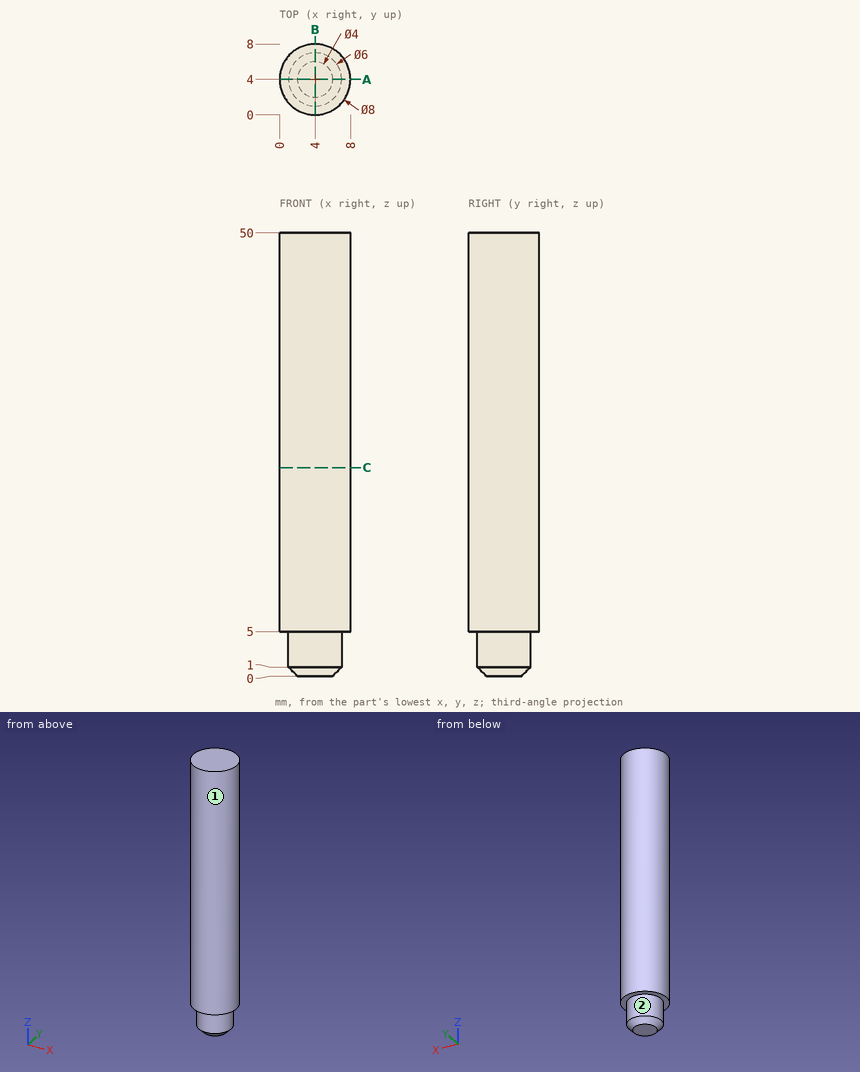
Geometry: see drawing. Coordinates: mm, zero at the bounding-box minimum. A direction names the side the tool comes from. Coordinates: 2 decimals unless noted, no trailing zeros. Loops run counter-clockwise (first coordinate to the right, second up) from the corner with the lowest first, then second, coordinate; pieces in that order, holes last. Notation, with made-up numbers: (-6.5, 33) - (32.5, 33) arc R24 ccw to (32.5, 48) - close; hole circle Ø9 at (-32, -3). An arc over 180 degrees is marked (long way). Put each result on its own line as item: value. Start each with the question number.
Q1. Set-up query: the marked faces 1 and 2. Return all of +Z, -Z, +X, -X, +Y, -Y with unobstructed straight access to the full face (end or side cutting, diameter ignored); none if empty.
Q2. Line query: line 1 (Z direction, x = 2, y = 6.75); line 2 (Y direction, x = 3.75, z = 31); line 3 (Y direction, x = 5.25, z = 22.5). Output: solid intervals per line, ascending.
Q3. Pin query (flat end, axial travel): pin 1 Ø1 at (x, z) = (2, 29.5) entering from -Y; pin 2 Ø2 at (x, z) = (6, 15.5) entering from -Y; pin 3 Ø3 at (y, z) = (6, 27.5) entering from -X. Return the tip coordinate at first contact, or that it passes through.
Q4. Cut plane A-A, the plane y = 4. Return loops of the section in (x, z), and give its area (3 significant figures).
Q5. Cut plane C-C, the plane z = 23.5. Return loops of the section in (x, y).
Filled sheet:
1. face 1: +Z, -Z
1. face 2: -Z
2. line 1: 5 to 50
2. line 2: 0.01 to 7.99
2. line 3: 0.2 to 7.8
3. pin 1: y = 0.29
3. pin 2: y = 0.13
3. pin 3: x = 0.03
4. outline: (0, 5) - (1, 5) - (1, 1) - (2, 0) - (6, 0) - (7, 1) - (7, 5) - (8, 5) - (8, 50) - (0, 50) - close
4. area: 389 mm²
5. outline: circle Ø8 at (4, 4)
